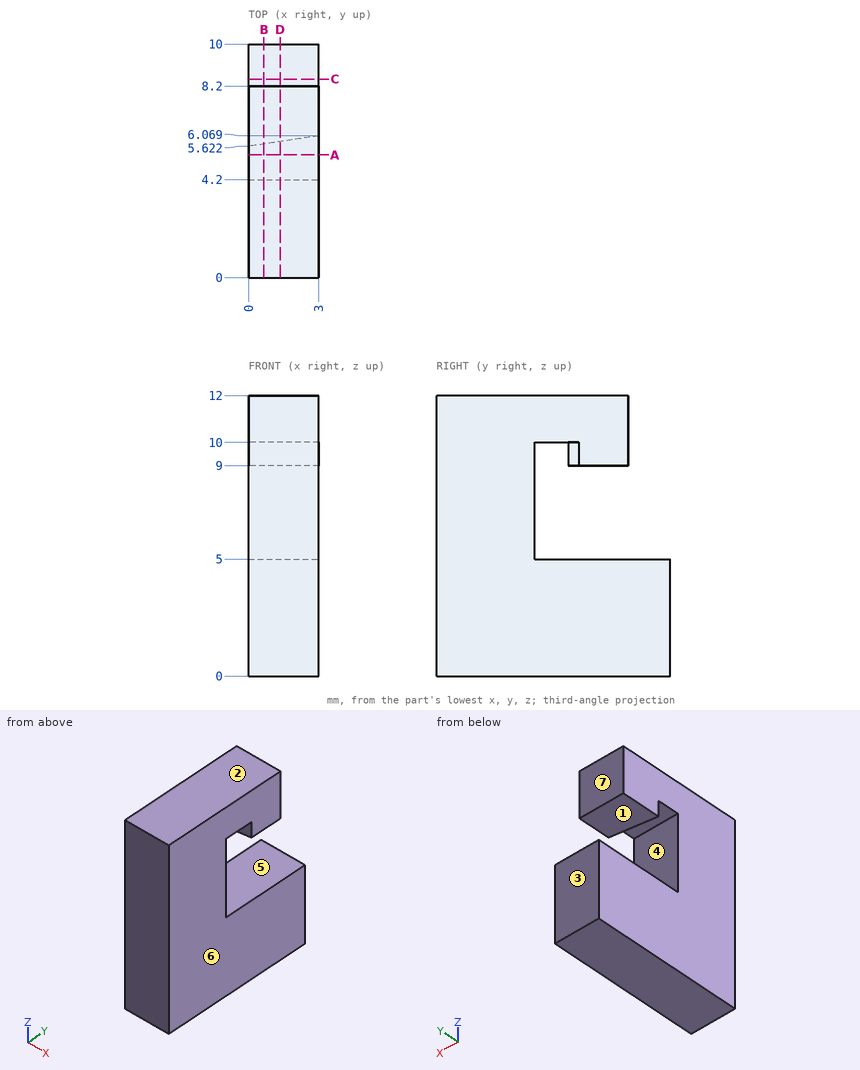
Here's the drawing with two shaded views (mm, measured from the low corner). I have some questions. A direction names the side the tool comes from. Coordinates: 2 decimals unless noted, no trailing zeros. Loops run counter-clockwise (first coordinate to the right, second up) from the corner with the lowest first, then second, coordinate; pieces in that order, holes last. Notation, with made-up numbers: (87.25, -16) -> (111.25, -16) arc R15 cw to (111.25, -6) -> close; hole circle Ø9 at (52, 26.25). An arc over 180 degrees is marked (long way). Put each result on its own line as item: value. Start each with the question number.
Q1. I want a section at C-C (y = 8.5). Write out the boundary of the cut face in (x, z).
Q2. I want a section at D-D (x = 1.35). Write out the boundary of the cut face in (y, z).
Q3. Thinking about a two-plate mould opening in Z: for the marked faces 1, 2, 3 and 4, which applies, pulls with the +Z half, pulls with the -Z half, needs draft (parallel to the pull), parting line crosses it, or undercut?
Q4. For the marked faces 5, 6 and 7, which set-ups out of +Z, -Z, +X, -X, +Y, -Y let a thin tool reach every point of the face, with its end or its side?
Q5. If I drill on line 1 (Z direction, x = 0.65, y = 4.25); line 2 (Z direction, x = 0.7, y = 6.25); line 3 (Y direction, x = 1.4, z = 6.75), over which ranges is the centre line in solid material (lowest first)? Write a range as [from, to].
Q6. I want a section at A-A (y = 5.25). Write out the boundary of the cut face in (x, z), plus the area to 3 significant figures.
Q7. I want a section at B-B (x = 0.65). Write out the boundary of the cut face in (y, z), plus the area to 3 significant figures.
Q8. I'm going to push a flat-ended pin straight in: P1, Ø0.9, axis at x = 2, z = 8.5, coming from the +Y side. Where does the tip first touch, or does it pass through?
Taken from the geometry:
1. outline: (0, 0) -> (3, 0) -> (3, 5) -> (0, 5) -> close
2. outline: (0, 0) -> (10, 0) -> (10, 5) -> (4.2, 5) -> (4.2, 10) -> (5.82, 10) -> (5.82, 9) -> (8.2, 9) -> (8.2, 12) -> (0, 12) -> close
3. face 1: undercut
3. face 2: pulls with the +Z half
3. face 3: needs draft
3. face 4: undercut
4. face 5: +X, -X, +Y
4. face 6: +Z, -Z, +X, +Y, -Y
4. face 7: +Z, +X, -X, +Y
5. line 1: z = [0, 5], [10, 12]
5. line 2: z = [0, 5], [9, 12]
5. line 3: y = [0, 4.2]
6. outline: (0, 0) -> (3, 0) -> (3, 5) -> (0, 5) -> close; (0, 10) -> (3, 10) -> (3, 12) -> (0, 12) -> close
6. area: 21.0 mm2
7. outline: (0, 0) -> (10, 0) -> (10, 5) -> (4.2, 5) -> (4.2, 10) -> (5.72, 10) -> (5.72, 9) -> (8.2, 9) -> (8.2, 12) -> (0, 12) -> close
7. area: 89.9 mm2
8. P1: stops at y = 4.2
